Input: part model. Units: mm. Frame: model coordinates. A direction names the side the tool comes from. Round coordinates to 2 decimals unless told otherwise and drop trailing zeros. Loops run counter-clockwise (first coordinate to the right, second up) from the corner with the lowest first, then second, coordinate; pieces in that order, holes last. Notation, with made-up numbers: (33.5, 51) - (76.5, 51) arc R9 ccw to (76.5, 55) - close; hole circle Ø9 at (14.25, 79.25). An arc over 180 degrees is marked (long way). One line per question, with ' | ' between items. Start each with the question number.
Item 1: Draft query along Y for faces 1 (the face through (-19, 5.556, 1)), 2 (the face through (-8.1, -8.13, 0.78)), 3 (the face through (8.72, -3.35, 0.78)). Return one class per face: pulls with the +Y half, pulls with the -Y half, needs draft (parallel to the pull), parting line crosses it, or undercut.
Item 2: Section A-A, the plane x = 0. Return loops of the section in (y, z).
Item 3: Material intervals for line 1 along Y through (x, z) = (0, 1); line 2 along Y through (x, z) = (-1.5, 0.45); line 3 along X through (y, z) = (8.75, 1.4), sorted ascending.
Item 4: Section D-D, the plane z = 1. Give the number of separate pieces and of enclosed holes in the cut face, plus the area to 3 significant figures.
Item 5: Set-up query: faces 4 (the face through (-5, 2, 1.588)), 5 (the face through (-18, 0, 1)), 6 (the face through (7.613, 7.82, 0.783)). Return all of +Z, -Z, +X, -X, +Y, -Y with unobstructed straight access to the full face (end or side cutting, diameter ignored); none if empty.
Item 6: First-contact query: pin 1 (1 mm diameter, centred on x = 2.5, y = 7.5, fed in from +Z). Flat tip, straight axial feed; report the tip coordinate or a pass-through.
Item 7: Section B-B, the plane x = -7. Return loops of the section in (y, z), plus the area to 3 significant figures.
Item 8: Section C-C, the plane y = 6.5. Return loops of the section in (x, z).
```python
from build123d import *

# Parameters (mm, degrees)
SKETCH1_R           = 1.7859375
BOSS_EXTRUDE1_DEPTH = 1.5875
FILLET1_R           = 3.175


with BuildPart() as part:
    # Sketch1 → Boss-Extrude1 (new body)
    with BuildSketch(Plane.XY):
        with BuildLine():
            Line((-14.492018868, 5.55625), (-19.446875, 5.55625))
            ThreePointArc((-19.446875, 5.55625), (-22.225, 2.778125), (-19.446875, 0))
            Line((-19.446875, 0), (-12.7, 0))
            ThreePointArc((-12.7, 0), (-12.267257994, -3.287001873), (-10.998522628, -6.35))
            ThreePointArc((-10.998522628, -6.35), (-6.11925064, -7.65739699), (-4.811853648, -2.778125003))
            ThreePointArc((-4.811853648, -2.778125003), (0.964832728, -5.47183807), (5.471838092, -0.964832608))
            ThreePointArc((5.471838092, -0.964832608), (8.369198647, -5.102692458), (12.507058463, -2.205331856))
            ThreePointArc((12.507058463, -2.205331856), (8.980256121, 8.980256121), (-2.205331856, 12.507058463))
            Line((-2.205331856, 12.507058463), (-11.976471281, 10.78414295))
            ThreePointArc((-11.976471281, 10.78414295), (-14.574868615, 8.815275161), (-14.492018868, 5.55625))
        make_face()
        with BuildLine():
            ThreePointArc((-1.274957479, 7.230643174), (-3.343887368, 8.679323478), (-1.895207064, 10.748253367))
            ThreePointArc((-1.895207064, 10.748253367), (7.717407604, 7.717407604), (10.748253367, -1.895207064))
            ThreePointArc((10.748253367, -1.895207064), (8.679323478, -3.343887368), (7.230643174, -1.274957479))
            ThreePointArc((7.230643174, -1.274957479), (5.19171057, 5.19171057), (-1.274957479, 7.230643174))
        make_face(mode=Mode.SUBTRACT)
        with Locations((-11.356221696, 7.266532758)):
            Circle(SKETCH1_R, mode=Mode.SUBTRACT)
        Circle(SKETCH1_R, mode=Mode.SUBTRACT)
        with Locations((-7.905188139, -4.5640625)):
            Circle(SKETCH1_R, mode=Mode.SUBTRACT)
    extrude(amount=BOSS_EXTRUDE1_DEPTH)

    # Fillet1
    fillet1_edges = [part.edges().sort_by_distance(p)[0] for p in [
        (-4.811853648, -2.778125003, 0.79375),
        (-12.7, 0, 0.79375),
        (-14.492018868, 5.55625, 0.79375),
        (5.471838092, -0.964832608, 0.79375),
    ]]
    fillet(fillet1_edges, radius=FILLET1_R)


solid = part.part
```
Return value:
1) face 1: pulls with the +Y half | face 2: pulls with the -Y half | face 3: undercut
2) outline: (-5.56, 0) - (-1.79, 0) - (-1.79, 1.59) - (-5.56, 1.59) - close; (1.79, 0) - (7.34, 0) - (7.34, 1.59) - (1.79, 1.59) - close; (10.91, 0) - (12.7, 0) - (12.7, 1.59) - (10.91, 1.59) - close
3) line 1: -5.56 to -1.79, 1.79 to 7.34, 10.91 to 12.7 | line 2: -5.35 to -0.97, 0.97 to 7.21, 10.81 to 12.61 | line 3: -14.61 to -12.35, -10.36 to -3.35, 6.52 to 9.2
4) separate pieces: 1 | enclosed holes: 4 | area: 374 mm2
5) face 4: +Z, +X, -X, +Y, -Y | face 5: +Z, -Z, -X, -Y | face 6: +Z, -Z
6) pin 1: through
7) outline: (-8.02, 0) - (-6.1, 0) - (-6.1, 1.59) - (-8.02, 1.59) - close; (-3.02, 0) - (11.66, 0) - (11.66, 1.59) - (-3.02, 1.59) - close | area: 26.4 mm2
8) outline: (-15.68, 0) - (-12.97, 0) - (-12.97, 1.59) - (-15.68, 1.59) - close; (-9.74, 0) - (3.41, 0) - (3.41, 1.59) - (-9.74, 1.59) - close; (8.77, 0) - (10.91, 0) - (10.91, 1.59) - (8.77, 1.59) - close
